Can you work these out from the model? Positions are in its coordinate system, mm. Face numbers are marked on the shaded views. A direction names the side the tool comes from. Coordinates: 2 decimals unless noted, no trailing zeros. Order: outer loops, then holes, each group sorted by start corner. A loop starts at its lowest first (then second) coordinate and runs counter-clockwise, first axis right, second up. Notation, with made-up numbers: (-35, 13) -> (-10, 13) arc R30 cw to (-10, 36) -> close; hole circle Ø9 at (8, -5). An arc over 180 degrees is marked (long way). Write item = value, one per line.
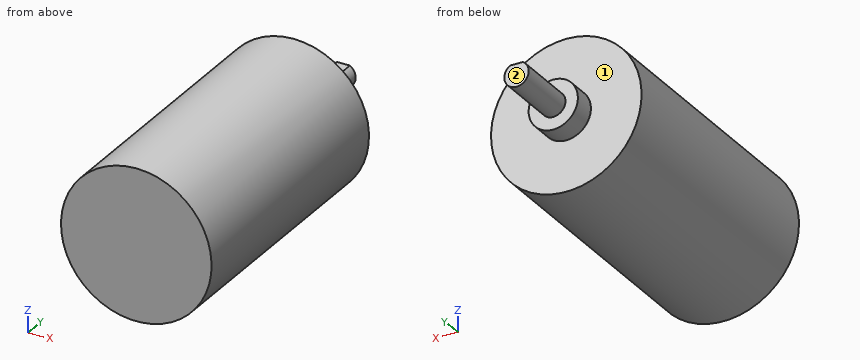
```python
from build123d import *

# Parameters (mm, degrees)
SKETCH1_R           = 185
BOSS_EXTRUDE1_DEPTH = 664
SKETCH2_R           = 60.5
BOSS_EXTRUDE2_DEPTH = 55
BOSS_EXTRUDE3_DEPTH = 155
SCALE1_SCALE        = 0.1


with BuildPart() as part:
    # Sketch1 → Boss-Extrude1 (new body)
    with BuildSketch(Plane(origin=(0, 0, 0), x_dir=(1, 0, 0), z_dir=(0, 1, 0))):
        with Locations(Location((0, 0, 0), (0, 0, 270))):
            Circle(SKETCH1_R)
    extrude(amount=BOSS_EXTRUDE1_DEPTH)

    # Sketch2 → Boss-Extrude2 (add)
    with BuildSketch(Plane(origin=(0, 664, 0), x_dir=(1, 0, 0), z_dir=(0, 1, 0))):
        with Locations(Location((0, 0, 0), (0, 0, 270))):
            Circle(SKETCH2_R)
    extrude(amount=BOSS_EXTRUDE2_DEPTH)

    # Sketch3 → Boss-Extrude3 (add)
    with BuildSketch(Plane(origin=(0, 719, 0), x_dir=(1, 0, 0), z_dir=(0, 1, 0))):
        with BuildLine():
            Line((0, -25.564167514), (15.699469395, -25.564167514))
            ThreePointArc((15.699469395, -25.564167514), (0, 30), (-15.699469395, -25.564167514))
            Line((-15.699469395, -25.564167514), (0, -25.564167514))
        make_face()
    extrude(amount=BOSS_EXTRUDE3_DEPTH)


with BuildPart() as part_1:
    # Scale1: scaled about (0, 337.854264359, -0.005518954)
    add(part.part.scale(SCALE1_SCALE).moved(Location((0, 304.068837923, -0.004967059))))


solid = part_1.part
```
Item 1: If I drill on probe 1 along X at (y, z) = (361.5, -0.5); probe 2 along Y at (x, z) = (12, -5.5); probe 3 along X at (y, z) = (345.5, -5.5), over which ranges is the centre line in solid material (lowest first)?
A:
probe_1 = -18.49 to 18.49
probe_2 = 304.07 to 370.47
probe_3 = -17.67 to 17.67
Item 2: I want a section at C-C, the plane z = 8. Please give me the cut outline in (x, y).
A:
outline = (-16.68, 304.07) -> (16.68, 304.07) -> (16.68, 370.47) -> (-16.68, 370.47) -> close
Item 3: I'm going to push flat-ended pins straight in: P1, Ø6, axis at x = 8, z = 4, coming from the +Y side; P2, Ø6, axis at y = 353.5, z = -12.5, coming from the +X side; P3, Ø3, axis at x = -10.5, z = -15, coming from the +Y side; P4, Ø10, axis at x = -2, y = 353.5, coming from the -Z side. Where does each tip first touch, or does it pass through?
A:
P1 = 375.97
P2 = 15.88
P3 = 370.47
P4 = -18.5
Item 4: For the marked faces 1 and 2, which set-ups out of +Z, -Z, +X, -X, +Y, -Y let a thin tool reach every point of the face, with its end or its side?
A:
face_1 = +Y
face_2 = +Z, -Z, +X, -X, +Y
Item 5: I want a section at D-D, the plane x = -4. Please give me the cut outline in (y, z), plus the area to 3 significant figures.
A:
outline = (304.07, -18.07) -> (370.47, -18.07) -> (370.47, -4.54) -> (375.97, -4.54) -> (375.97, 4.53) -> (370.47, 4.53) -> (370.47, 18.06) -> (304.07, 18.06) -> close
area = 2,450 mm2
Item 6: I want a section at B-B, the plane y = 326. Please give me the cut outline in (x, z).
A:
outline = circle Ø37 at (0, 0)
Item 7: I want a section at A-A, the plane x = 0. Please give me the cut outline in (y, z), plus the area to 3 significant figures.
A:
outline = (304.07, -18.5) -> (370.47, -18.5) -> (370.47, -6.05) -> (375.97, -6.05) -> (375.97, -3) -> (391.47, -3) -> (391.47, 2.55) -> (375.97, 2.55) -> (375.97, 6.05) -> (370.47, 6.05) -> (370.47, 18.5) -> (304.07, 18.5) -> close
area = 2,610 mm2
